Check sheet for the modelled part. Datum: model origin and axes. Units: mm. Face numbers are marked on the shaded views. Round coordinates to 2 decimals unless told otherwise and drop trailing zeros. Write each loop counter-clockwise with the first axis right and the second up, starting at its lowest first coordinate (ties: lowest second). Pieces come first, ordered by that corner, then holes. Notation, with made-up numbers: (86, 58) -> (102, 58) arc R22 cw to (102, 93) -> close; hole circle Ø2 at (-15, 49). An arc over 180 degrees is marked (long way). One line per item, written item: value.
from build123d import *


with BuildPart() as part:
    # Sketch1 → Revolve1 (revolve)
    with BuildSketch(Plane.XY, mode=Mode.PRIVATE) as revolve1_sk:
        with BuildLine():
            Line((0, 0), (0, 15))
            Line((0, 15), (-16, 15))
            Line((-16, 15), (-16, 11.5))
            Line((-16, 11.5), (-12.5, 11.5))
            Line((-12.5, 11.5), (-12.5, 8.5))
            Line((-12.5, 8.5), (-7.5, 8.5))
            Line((-7.5, 8.5), (-7.5, 6.35483871))
            Line((-7.5, 6.35483871), (-15, 6.35483871))
            Line((-15, 6.35483871), (-21.131764452, 11.5))
            Line((-21.131764452, 11.5), (-24.544040459, 11.5))
            ThreePointArc((-24.544040459, 11.5), (-25.829615679, 11.032088886), (-26.513655966, 9.847296355))
            Line((-26.513655966, 9.847296355), (-28.25, 0))
            Line((-28.25, 0), (0, 0))
        make_face()
    revolve(revolve1_sk.sketch.rotate(Axis((0, 0, 0), (0, -1, 0)), 270), axis=Axis((0, 0, 0), (0, -1, 0)))


solid = part.part
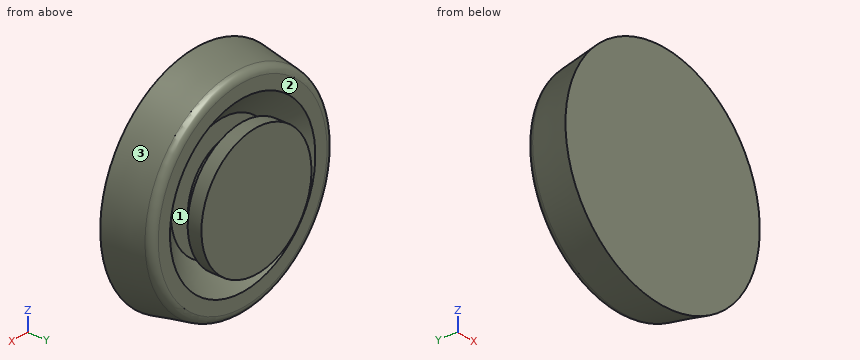
Item 1: Depth check by flat-ended pin: pin 1 (12 mm diameter, centred on x = 20.5, z = -17, fed in from +Y); pin 2 (5 mm diameter, centred on y = 8.5, z = 15, fed in from -X); pin 3 (5 mm diameter, centred on x = -21, y = 2, fed in from +Z). Enter the tip coordinate at first touch or a pass-through.
Result set:
pin 1: y = 11.5
pin 2: x = -23.74
pin 3: z = 20.96
Item 2: Sectioned sample at B-B (x = 0). Enter the section's corners in (y, z), then the cut area to 3 significant figures.
Result set:
outline: (0, -28.25) -> (9.85, -26.51) arc R2 ccw to (11.5, -24.54) -> (11.5, -21.13) -> (6.35, -15) -> (6.35, -7.5) -> (8.5, -7.5) -> (8.5, -12.5) -> (11.5, -12.5) -> (11.5, -16) -> (15, -16) -> (15, 16) -> (11.5, 16) -> (11.5, 12.5) -> (8.5, 12.5) -> (8.5, 7.5) -> (6.35, 7.5) -> (6.35, 15) -> (11.5, 21.13) -> (11.5, 24.54) arc R2 ccw to (9.85, 26.51) -> (0, 28.25) -> close
area: 659 mm^2
Item 3: Sectioned sample at D-D (y = 2.5). Enter the section's corners in (x, z).
Result set:
outline: circle Ø55.62 at (0, 0)
Item 4: Sectioned sample at C-C (y = 13.5). Enter the section's corners in (x, z).
Result set:
outline: circle Ø32 at (0, 0)
Item 5: Release check for a two-part mould opening along X. For the marked faces 1, 2 and 3 record: pulls with the +X half, pulls with the -X half, needs draft (parallel to the pull), parting line crosses it, or undercut.
Result set:
face 1: undercut
face 2: needs draft
face 3: parting line crosses it
Item 6: Sectioned sample at A-A (z = 0). Enter the section's corners in (x, y), then the cut area to 3 significant figures.
Result set:
outline: (-28.25, 0) -> (28.25, 0) -> (26.51, 9.85) arc R2 ccw to (24.54, 11.5) -> (21.13, 11.5) -> (15, 6.35) -> (7.5, 6.35) -> (7.5, 8.5) -> (12.5, 8.5) -> (12.5, 11.5) -> (16, 11.5) -> (16, 15) -> (-16, 15) -> (-16, 11.5) -> (-12.5, 11.5) -> (-12.5, 8.5) -> (-7.5, 8.5) -> (-7.5, 6.35) -> (-15, 6.35) -> (-21.13, 11.5) -> (-24.54, 11.5) arc R2 ccw to (-26.51, 9.85) -> close
area: 659 mm^2
Item 7: Material ranges on line 1 along X through (y, z) = (7.5, -3); line 2 along Y through (x, z) = (1, 13); line 3 along X through (y, z) = (10.5, 4.5), recorded low to high.
Result set:
line 1: -26.76 to -16.09, -6.87 to 6.87, 16.09 to 26.76
line 2: 0 to 6.35, 11.5 to 15
line 3: -25.89 to -19.43, -11.66 to 11.66, 19.43 to 25.89
